from build123d import *

# Parameters (mm, degrees)
F0_R     = 4.7625
F1_DEPTH = 63.5
F2_R     = 8.89
F3_DEPTH = 12.7
F5_DEPTH = 9.5377


with BuildPart() as f1:
    # F0 (on Top) → F1 (new body)
    with BuildSketch(Plane.XY):
        Circle(F0_R)
    extrude(amount=-F1_DEPTH)

    # F2 (on Top) → F3 (join)
    with BuildSketch(Plane.XY):
        Circle(F2_R)
    extrude(amount=F3_DEPTH)

    # F4 (on face) → F5 (cut)
    with BuildSketch(Plane.XY.offset(12.7)):
        Polygon((5.293086, -3.055965), (5.293086, 3.055965), (0, 6.111929), (-5.293086, 3.055965), (-5.293086, -3.055965), (0, -6.111929), align=None)
    extrude(amount=-F5_DEPTH, mode=Mode.SUBTRACT)


solid = f1.part
Source: CAD feature listing. Evaluate the final solid. Frame: model axes, mm. A direction names the side the tool comes from. Give positions to 0.01 mm unless a question says otherwise; leave off trailing zeros. Write each loop counter-clockwise with the first axis right and the second up, starting at its lowest first coordinate (ties: lowest second). Pieces come first, ordered by that corner, then holes. Notation, with made-up numbers: (7.5, -0.5) -> (41.5, -0.5) arc R33 ccw to (41.5, 32.5) -> close; hole circle Ø2 at (25.5, 27.25). An arc over 180 degrees is marked (long way). Return JSON: item names as keys, results as strings. Group by question number.
1. Section A-A, the plane x = -2. Output: boundary loops of the cut face in (y, z), then the cut area to 3 significant figures.
2. Material intervals for line 1 (Z direction, x = 4.5, y = -5); line 2 (Z direction, x = -0.25, y = -1.5); line 3 (Y direction, x = 1.25, z = -53), sorted ascending. Write a range as from..to.
3. Section B-B, the plane y = 1.5. Output: boundary loops of the cut face in (x, z).
4. Access query for faces 4 (the face through (4, -4, 0)), 5 (the face through (-1.93, -8.68, 6.26)), 6 (the face through (-2.684, -4.563, 7.998)). Directions: +Z, -Z, +X, -X, +Y, -Y. A direction counts if a zero-diameter tool reaches every point of the face in a straight line with its end or side. Return the directions, or none.
5. Mould query, pull axis X, two halves, no side actions, for faces 1 (the face through (4, 4, 12.7)), 2 (the face through (-5.293, 0, 8)), 3 (the face through (-3.78, -2.9, -31.31)). Classes: +X half, -X half, draft (parallel to the pull), parting line (faces both ways), or undercut.
6. Section C-C, the plane z = -12. Output: boundary loops of the cut face in (x, y) (1 decimal), then the cut area to 3 significant figures.
7. Section D-D, the plane x = 6. Output: boundary loops of the cut face in (y, z), then the cut area to 3 significant figures.
8. Pin query (flat end, axial travel): pin 1 Ø5 at (x, z) = (6.5, -37.5) entering from -Y; pin 2 Ø3 at (x, y) = (-1, 1) entering from +Z; pin 3 Ø5 at (x, y) = (-7, -4.5) entering from -Z; pin 4 Ø5 at (y, z) = (0.5, 9) entering from -X. Return the tip coordinate at first contact, or that it passes through.
Determined:
{
 "1": {"outline": "(-8.66, 0) -> (-4.32, 0) -> (-4.32, -63.5) -> (4.32, -63.5) -> (4.32, 0) -> (8.66, 0) -> (8.66, 12.7) -> (4.96, 12.7) -> (4.96, 3.16) -> (-4.96, 3.16) -> (-4.96, 12.7) -> (-8.66, 12.7) -> close", "area": "674 mm2"},
 "2": {"line 1": "z = 0..12.7", "line 2": "z = -63.5..3.16", "line 3": "y = -4.6..4.6"},
 "3": {"outline": "(-8.76, 0) -> (-4.52, 0) -> (-4.52, -63.5) -> (4.52, -63.5) -> (4.52, 0) -> (8.76, 0) -> (8.76, 12.7) -> (5.29, 12.7) -> (5.29, 3.16) -> (-5.29, 3.16) -> (-5.29, 12.7) -> (-8.76, 12.7) -> close"},
 "4": {"face 4": "-Z", "face 5": "+Z, -Z", "face 6": "+Z"},
 "5": {"face 1": "draft", "face 2": "undercut", "face 3": "parting line"},
 "6": {"outline": "circle Ø9.5 at (0, 0)", "area": "71.3 mm2"},
 "7": {"outline": "(-6.56, 0) -> (6.56, 0) -> (6.56, 12.7) -> (-6.56, 12.7) -> close", "area": "167 mm2"},
 "8": {"pin 1": "stops at y = -2.58", "pin 2": "stops at z = 3.16", "pin 3": "stops at z = 0", "pin 4": "stops at x = -8.89"}
}
